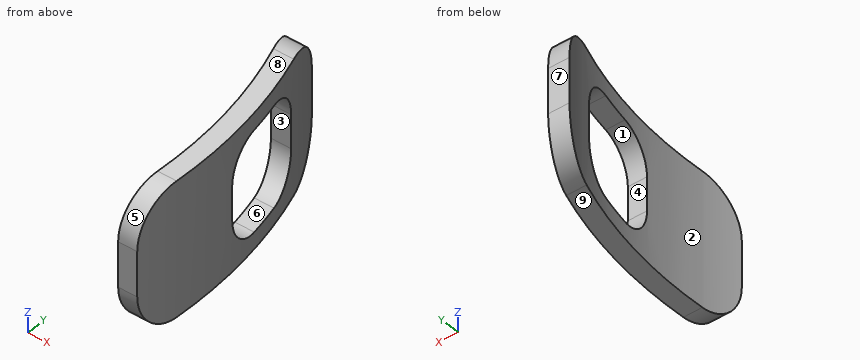
```python
from build123d import *

# Parameters (mm, degrees)
BOSS_EXTRUDE2_DEPTH     = 609.6
FILLET1_R               = 203.2
CUT_EXTRUDE1_DEPTH      = 2530.244458167
CUT_EXTRUDE1_DEPTH_BACK = 2530.244458167


with BuildPart() as part:
    # Sketch1 → Boss-Extrude2 (new body)
    with BuildSketch(Plane.XY):
        with BuildLine():
            Line((1903.109301748, 1003.3), (2003.058558405, 1003.3))
            ThreePointArc((2003.058558405, 1003.3), (2202.497656801, 409.705443199), (2229.852387132, -215.9))
            Line((2229.852387132, -215.9), (2140.519351559, -215.9))
            ThreePointArc((2140.519351559, -215.9), (2111.716205237, 411.206241365), (1903.109301748, 1003.3))
        make_face()
    extrude(amount=BOSS_EXTRUDE2_DEPTH)

    # Fillet1
    fillet1_edges = [part.edges().sort_by_distance(p)[0] for p in [
        (2185.185869346, -215.9, 609.6),
        (2185.185869346, -215.9, 0),
        (1953.083930077, 1003.3, 0),
        (1953.083930077, 1003.3, 609.6),
    ]]
    fillet(fillet1_edges, radius=FILLET1_R)

    # Sketch2 → Cut-Extrude1 (cut, two sides: drawn at the far end of the back side and taken through both)
    with BuildSketch(Plane(origin=(0, 0, 0), x_dir=(0, 0, -1), z_dir=(1, 0, 0)).offset(-CUT_EXTRUDE1_DEPTH_BACK)):
        with BuildLine():
            Line((-381, 317.5), (-228.6, 317.5))
            ThreePointArc((-228.6, 317.5), (-120.836926547, 362.136926547), (-76.2, 469.9))
            Line((-76.2, 469.9), (-76.2, 622.3))
            ThreePointArc((-76.2, 622.3), (-120.836926547, 730.063073453), (-228.6, 774.7))
            Line((-228.6, 774.7), (-381, 774.7))
            ThreePointArc((-381, 774.7), (-488.763073453, 730.063073453), (-533.4, 622.3))
            Line((-533.4, 622.3), (-533.4, 469.9))
            ThreePointArc((-533.4, 469.9), (-488.763073453, 362.136926547), (-381, 317.5))
        make_face()
    extrude(amount=CUT_EXTRUDE1_DEPTH + CUT_EXTRUDE1_DEPTH_BACK, mode=Mode.SUBTRACT)


solid = part.part
```
Here's how the part is built. I have some questions about the finished solid (model axes, mm). Face numbers are marked on the shaded views. A direction names the side the tool comes from. Coordinates: 2 decimals unless noted, no trailing zeros. Write each loop counter-clockwise with the first axis right and the second up, starting at its lowest first coordinate (ties: lowest second). Pieces come first, ordered by that corner, then holes. Notation, with made-up numbers: (-19, -4.75) - (-15, -4.75) arc R29 cw to (-15, 16.25) - close; hole circle Ø4 at (64.5, -35.75). An arc over 180 degrees is marked (long way). One line per item, written item: value.
1) On a 3-axis mill with a long thin cutter (end or side, diameter ignored), from which of +Z, -Z, +X, -X, +Y, -Y can I reach the whole of each face in a straight line? I mean the marked faces 1, 2, 3, 4 and 5. Say none if no direction works.
Model answer:
face 1: +X, -X
face 2: +Z, -Z, -X
face 3: +X, -X, -Y
face 4: +X, -X, +Y
face 5: +Z, +X, -X, -Y
2) Suppose I cut it at D-D on y = -87. Write out the boundary of the cut face in (x, z), and give its area (3 significant figures).
Model answer:
outline: (2149.62, 14.07) - (2238.59, 14.07) - (2238.59, 595.53) - (2149.62, 595.53) - close
area: 51,700 mm²
3) Suppose I cut it at C-C on x = 1949.5. Write out the boundary of the cut face in (y, z).
Model answer:
outline: (909.88, 32.21) arc R203.2 ccw to (1003.3, 203.2) - (1003.3, 406.4) arc R203.2 ccw to (909.88, 577.39) - close
4) We'd pull the mould along Z, two halves only. Please class the marked faces 6, 7, 8 and 9: pulls with the +Z half, pulls with the -Z half, needs draft (parallel to the pull), parting line crosses it, or undercut.
Model answer:
face 6: undercut
face 7: needs draft
face 8: pulls with the +Z half
face 9: pulls with the -Z half
5) Suppose I cut it at A-A on z = 107.5. Write out the boundary of the cut face in (x, y).
Model answer:
outline: (1915.54, 979.35) arc R2151.38 cw to (2029.15, 714.82) - (2123.18, 714.82) arc R2240.28 ccw to (2014.88, 979.35) - close; (2118.02, 377.38) arc R2151.38 cw to (2142.8, -191.95) - (2232.04, -191.95) arc R2240.28 ccw to (2208.27, 377.38) - close
6) I'm going to push flat-ended pins straight in: P1, Ø8, axis at y = -36, z = 260, coming from the -X side; P2, Ø1, axis at x = 2193, y = -27.5, coming from the +Z side. Where does each tip first touch, or does it pass through?
Model answer:
P1: stops at x = 2151.01
P2: stops at z = 609.1
7) Suppose I cut it at B-B on y = 737.5. Write out the boundary of the cut face in (x, z).
Model answer:
outline: (2021.02, 0) - (2115.41, 0) - (2115.41, 128.83) - (2021.02, 128.83) - close; (2021.02, 480.77) - (2115.41, 480.77) - (2115.41, 609.6) - (2021.02, 609.6) - close
8) I need wall thicknesses on line 1 along Z through (x, y) = (2164, 485); line 2 along Y through (x, z) = (2194.5, 380); line 3 along X through (y, z) = (216, 315.5). Which ranges of each line are inside material? Lowest first, please.
Model answer:
line 1: z = 0 to 76.2, 533.4 to 609.6
line 2: y = -215.9 to 317.5
line 3: x = 2140.51 to 2229.84
